Autodesk Inventor part; units mm, degrees
ref_plane "YZ Plane" through (0, 0, 0) normal (1, 0, 0) x (0, 1, 0)
ref_plane "XZ Plane" through (0, 0, 0) normal (0, 1, 0) x (-1, 0, 0)
ref_plane "XY Plane" through (0, 0, 0) normal (0, 0, 1) x (1, 0, 0)
sketch "main" plane through (0, 0, 0) normal (0, 0, 1) x (1, 0, 0)
  circle A0 centre (-18.8876, -3.9215) radius 2.0828
  arc A1 (-24.8429, -6.1253) -> (-18.8884, -10.2715) centre (-18.8876, -3.9215) ccw
  line L0 (5.8565, 45.4052) -> (-28.0879, 4.9518)
  circle A2 centre (9.8531, -3.9215) radius 2.1844
  line L1 (-18.8884, -10.2715) -> (35.2523, -10.2783)
  line L2 (9.8472, 18.301) -> (9.8489, 11.9535)
  arc A3 (9.8489, 11.9535) -> (19.3764, 2.4311) centre (19.3739, 11.9561) ccw
  circle A4 centre (9.8531, 34.1785) radius 2.1844
  line L3 (35.2514, 2.4354) -> (19.3764, 2.4311)
  arc A5 (35.2523, -10.2783) -> (35.2514, 2.4354) centre (35.2531, -3.9215) ccw
  circle A6 centre (35.2531, 34.1785) radius 2.1844
  arc A7 (35.2531, 27.8285) -> (36.6181, 40.3801) centre (35.2531, 34.1785) ccw
  circle A8 centre (35.2531, -3.9215) radius 2.1844
  line L4 (-28.3606, 3.3804) -> (-24.8429, -6.1253)
  line L5 (19.3722, 27.8285) -> (35.2531, 27.8285)
  arc A9 (19.3722, 27.8285) -> (9.8472, 18.301) centre (19.3722, 18.3035) ccw
  circle A10 centre (-14.2094, 14.0824) radius 2.0828
  arc A11 (-28.0879, 4.9518) -> (-28.3606, 3.3804) centre (-26.8718, 3.9314) ccw
  circle A12 centre (-4.1684, 26.0488) radius 2.0828
  line L6 (-4.1684, 26.0488) -> (-14.2094, 14.0824)
  line L7 (8.9712, 46.4651) -> (36.6181, 40.3801)
  arc A13 (8.9712, 46.4651) -> (5.8565, 45.4052) centre (8.2887, 43.3643) ccw
  point P0 (9.379, 13.4106)
  point P1 (9.8514, 2.4285)
  point P2 (9.8446, 27.8285)
  dimension "d0" = 4.1656
  dimension "d1" = 12.7
  dimension "d6" = 9.525
  dimension "d8" = 4.1656
  dimension "d9" = 1.5875
  dimension "d14" = 4.1656
  dimension "d15" = 15.621
  dimension "d17" = 3.175
sketch "Sketch1" plane through (0, 0, 0) normal (0, 1, 0) x (-1, 0, 0)
  circle A0 centre (-54.1407, -38.1) radius 2.0828
  arc A1 (-60.096, -40.3039) -> (-54.1415, -44.45) centre (-54.1407, -38.1) ccw
  line L0 (-29.3966, 11.2266) -> (-63.341, -29.2268)
  circle A2 centre (-25.4, -38.1) radius 2.1844
  line L1 (-54.1415, -44.45) -> (-0.0008, -44.4568)
  line L2 (-25.406, -15.8776) -> (-25.4043, -22.225)
  arc A3 (-25.4043, -22.225) -> (-15.8767, -31.7474) centre (-15.8793, -22.2224) ccw
  circle A4 centre (-25.4, 0) radius 2.1844
  line L3 (-0.0017, -31.7432) -> (-15.8767, -31.7474)
  arc A5 (-0.0008, -44.4568) -> (-0.0017, -31.7432) centre (0, -38.1) ccw
  circle A6 centre (0, 0) radius 2.1844
  arc A7 (0, -6.35) -> (1.3649, 6.2016) centre (0, 0) ccw
  circle A8 centre (0, -38.1) radius 2.1844
  line L4 (-63.6138, -30.7981) -> (-60.096, -40.3039)
  line L5 (-15.881, -6.35) -> (0, -6.35)
  arc A9 (-15.881, -6.35) -> (-25.406, -15.8776) centre (-15.881, -15.875) ccw
  circle A10 centre (-49.4625, -20.0961) radius 2.0828
  arc A11 (-63.341, -29.2268) -> (-63.6138, -30.7981) centre (-62.1249, -30.2472) ccw
  circle A12 centre (-39.4215, -8.1298) radius 2.0828
  line L6 (-39.4215, -8.1298) -> (-49.4625, -20.0961)
  line L7 (-26.2819, 12.2866) -> (1.3649, 6.2016)
  arc A13 (-26.2819, 12.2866) -> (-29.3966, 11.2266) centre (-26.9644, 9.1858) ccw
extrude "Extrusion1" add sketch "Sketch1" along normal blind 1.5875
properties part number "funel_gusset" material "Acetal Resin, White"
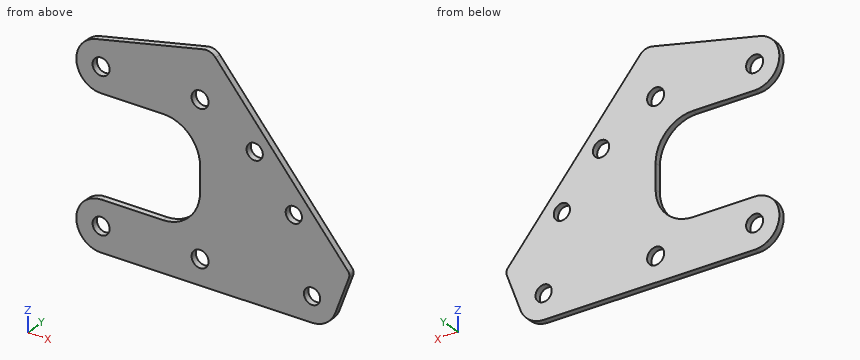
The model under review builds one solid part; all positions refer to its coordinate system, in mm. Give positions to 0.01 mm unless a question says otherwise; leave off trailing zeros. Order: outer loops, then holes, each group sorted by start corner. A loop starts at its lowest first (then second) coordinate and runs counter-clockwise, first axis right, second up. Notation, with made-up numbers: (27, 51) - (71, 51) arc R23 cw to (71, 70) - close; hole circle Ø7 at (71, -39.5). An arc over 180 degrees is marked (long way). Use CSV: the item, a comma, the result in double quotes. Start each with the question number.
Q1. To check wall thickness, follow line 1 along Z through (x, y) = (26, 1.45); line 2 along Z through (x, y) = (0, 0.7); line 3 along Z through (x, y) = (14, 0.8). State the ranges of each line that lie inside material, in increasing order. Write a range as [from, to].
Q2. We need section A-A, the plane x = 50. Write out the cut boundary in (y, z), and give its area (3 significant figures).
Q3. We need section C-C, the plane y = 0.6. State how many separate pieces and enclosed holes the cut face has, and give its area (3 significant figures).
Q4. We need section B-B, the plane z = 0. Write out the cut boundary in (x, y), and give its area (3 significant figures).
Q5. We need section D-D, the plane z = -38.1. Write out the cut boundary in (x, y), and give its area (3 significant figures).
Q6. Clearance check with flat-ended pins moving along their axes: pin 1 Ø3.5 at (x, z) = (54.14, -38.1) entering from -Y; pin 2 Ø0.5 at (y, z) = (1, -20) entering from -X; pin 3 Ø0.8 at (x, y) = (10.5, 1) entering from +Z. State where each tip first meets the part, or that it passes through.
Outcome:
1,line 1,"z = [-44.45, -40.2], [-36, -2.1], [2.1, 12.22]"
1,line 2,"z = [-44.46, -40.28], [-35.92, -31.74], [-6.35, -2.18], [2.18, 6.5]"
1,line 3,"z = [-44.46, -31.75], [-6.35, 9.58]"
2,outline,"(0, -44.45) - (1.59, -44.45) - (1.59, -22.11) - (0, -22.11) - close; (0, -18.08) - (1.59, -18.08) - (1.59, -13.33) - (0, -13.33) - close"
2,area,"43.0 mm^2"
3,separate pieces,"1"
3,enclosed holes,"7"
3,area,"2,180 mm^2"
4,outline,"(-6.35, 0) - (-2.18, 0) - (-2.18, 1.59) - (-6.35, 1.59) - close; (2.18, 0) - (23.22, 0) - (23.22, 1.59) - (2.18, 1.59) - close; (27.58, 0) - (38.82, 0) - (38.82, 1.59) - (27.58, 1.59) - close"
4,area,"57.8 mm^2"
5,outline,"(-6.36, 0) - (-2.18, 0) - (-2.18, 1.59) - (-6.36, 1.59) - close; (2.18, 0) - (23.22, 0) - (23.22, 1.59) - (2.18, 1.59) - close; (27.58, 0) - (52.06, 0) - (52.06, 1.59) - (27.58, 1.59) - close; (56.22, 0) - (60.91, 0) - (60.91, 1.59) - (56.22, 1.59) - close"
5,area,"86.3 mm^2"
6,pin 1,"passes through"
6,pin 2,"stops at x = 25.4"
6,pin 3,"stops at z = 8.9"
